Input: part model. Units: mm. Frame: model coordinates. Face numbers are marked on the shaded views. A direction names the side the tool comes from. Give positions to 0.01 mm unless a question says otherwise; leave off trailing zeros. Loops run counter-clockwise (first coordinate to the right, second up) from the corner with the lowest first, then second, coordinate; pieces in that order, holes last. Notation, with made-up numbers: M -30,-22 L -20,-22 A19 ccw -20,14 Z; hole C 64.25,80 d3. An arc over 180 degrees is marked long. One line per item, written item: value. Start each with the question number.
(1) Access query for the marked faces 1 and 2. Directions: +Z, -Z, +X, -X, +Y, -Y. A direction counts if a zero-diameter tool reaches every point of the face in a straight line with its end or side. Return the directions, or none.
(2) Ray query, line 1 along Y through (x, z) = (27, -2.5); line 2 along Z through (x, y) = (20, 14.9); line 3 along X through (y, z) = (8.5, 1.75). Return the intervals inside material, ascending. Write a range as from..to.
(3) Section D-D on x = 13.5. Output: boundary loops of the cut face in (y, z).
(4) Section A-A on z = 0. Output: boundary loops of the cut face in (x, y), plus the area to 3 significant figures.
(5) Section B-B on x = 20. Output: boundary loops of the cut face in (y, z).
(6) Pull-direction query (Y, two-part tool) for the marked faces 3, 4, 5 and 6; classes: released by +Y, released by -Y, zero draft, split by the parting line, or undercut.
(7) Pin query (flat end, axial travel): P1, Ø1.2, axis at y = 11.5, z = -1, coming from the +X side; P2, Ø3, axis at y = 9.5, z = -1.5, coming from the -X side; P3, Ø10, axis at x = 12, y = 12, coming from the +Z side; P4, Ø1.5, axis at y = -12.5, z = 1.5, coming from the -X side. Return the tip coordinate at first contact, or that it passes through.
(8) Section C-C on z = -2.75. Output: boundary loops of the cut face in (x, y).
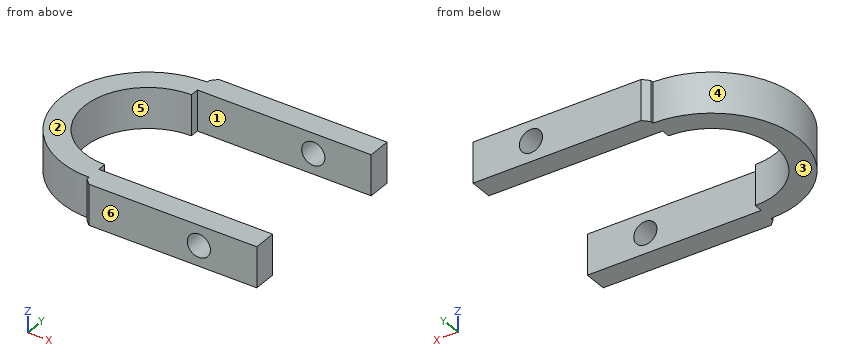
```python
from build123d import *

# Parameters (mm, degrees)
BOX001_W               = 30
BOX001_H               = 25
BOX001_DEPTH           = 7
CYLINDER002_R          = 2
CYLINDER002_DEPTH      = 40
CYLINDER002_ROLL_ANGLE = -90
CYLINDER_R             = 11
CYLINDER_DEPTH         = 7
CYLINDER001_R          = 15
CYLINDER001_DEPTH      = 7
BOX_W                  = 30
BOX_H                  = 33
BOX_DEPTH              = 7
CHAMFER_SIZE           = 1


with BuildPart() as cube001:
    # Box001 → Box001 (new body)
    with BuildSketch(Plane(origin=(0, -12.5, -3.5), x_dir=(1, 0, 0), z_dir=(0, 0, 1))):
        with Locations((15, 12.5)):
            Rectangle(BOX001_W, BOX001_H)
    extrude(amount=BOX001_DEPTH)


with BuildPart() as screw:
    # Cylinder002 → Cylinder002 (new body)
    with BuildSketch(Plane.XY):
        Circle(CYLINDER002_R)
    extrude(amount=CYLINDER002_DEPTH)


with BuildPart() as screw_1:
    # Cylinder002 roll: moved
    add(screw.part.rotate(Axis((0, 0, 0), (1, 0, 0)), CYLINDER002_ROLL_ANGLE))


with BuildPart() as screw_2:
    # Cylinder002 placement: moved
    add(screw_1.part.moved(Location((20, -20, 0))))


with BuildPart() as negative_fusion:
    # Cylinder → Cylinder (new body)
    with BuildSketch(Plane.XY.offset(-3.5)):
        Circle(CYLINDER_R)
    extrude(amount=CYLINDER_DEPTH)

    # Fusion001: union Cube001, Screw
    add(cube001.part)
    add(screw_2.part)


with BuildPart() as bearingouter:
    # Cylinder001 → Cylinder001 (new body)
    with BuildSketch(Plane.XY.offset(-3.5)):
        Circle(CYLINDER001_R)
    extrude(amount=CYLINDER001_DEPTH)


with BuildPart() as chamfer_body:
    # Box → Box (new body)
    with BuildSketch(Plane(origin=(0, -16.5, -3.5), x_dir=(1, 0, 0), z_dir=(0, 0, 1))):
        with Locations((15, 16.5)):
            Rectangle(BOX_W, BOX_H)
    extrude(amount=BOX_DEPTH)

    # Fusion: union BearingOuter
    add(bearingouter.part)

    # Cut: cut Negative Fusion
    add(negative_fusion.part, mode=Mode.SUBTRACT)

    # Chamfer
    chamfer_edges = [chamfer_body.edges().sort_by_distance(p)[0] for p in [
        (0, -16.5, 0),
        (0, 16.5, 0),
    ]]
    chamfer(chamfer_edges, length=CHAMFER_SIZE)


solid = chamfer_body.part
```
Output values:
1. face 1: +Z, -Z, +X
1. face 2: +Z, +X, -X, +Y, -Y
2. line 1: y = -16.5..-12.5, 12.5..16.5
2. line 2: z = -3.5..-2, 2..3.5
2. line 3: x = -12.36..-6.98
3. outline: M -16.5,-3.5 L -12.5,-3.5 L -12.5,3.5 L -16.5,3.5 Z; M 12.5,-3.5 L 16.5,-3.5 L 16.5,3.5 L 12.5,3.5 Z
4. outline: M 0,-15.5 L 1,-16.5 L 18,-16.5 L 18,-12.5 L 0,-12.5 L 0,-11 A11 cw 0,11 L 0,12.5 L 18,12.5 L 18,16.5 L 1,16.5 L 0,15.5 L 0,15 A15 ccw 0,-15 Z; M 22,-16.5 L 30,-16.5 L 30,-12.5 L 22,-12.5 Z; M 22,12.5 L 30,12.5 L 30,16.5 L 22,16.5 Z
4. area: 370 mm²
5. outline: M -16.5,-3.5 L -12.5,-3.5 L -12.5,-2 L -16.5,-2 Z; M -16.5,2 L -12.5,2 L -12.5,3.5 L -16.5,3.5 Z; M 12.5,-3.5 L 16.5,-3.5 L 16.5,-2 L 12.5,-2 Z; M 12.5,2 L 16.5,2 L 16.5,3.5 L 12.5,3.5 Z
6. face 3: zero draft
6. face 4: split by the parting line
6. face 5: undercut
6. face 6: released by -Y
7. P1: stops at x = 0
7. P2: stops at x = -12.69
7. P3: stops at z = 3.5
7. P4: stops at x = -9.32
8. outline: M 0,-15.5 L 1,-16.5 L 30,-16.5 L 30,-12.5 L 0,-12.5 L 0,-11 A11 cw 0,11 L 0,12.5 L 30,12.5 L 30,16.5 L 1,16.5 L 0,15.5 L 0,15 A15 ccw 0,-15 Z
